Geometry: final body of the model. Coordinates: model frame, mm. A direction names the side the tool comes from. Coordinates: 2 decimals unless noted, no trailing zeros. Write each loop counter-clockwise with the first axis right and the second up, starting at its lowest first coordinate (ties: lowest second). Pieces come first, ordered by that corner, then holes. Notation, with made-up numbers: (11, 9.25) -> (48, 9.25) arc R20 cw to (48, 22.25) -> close; hole circle Ø11 at (10.5, -18.75). An arc over 180 degrees is marked (long way). One line per item, written item: value. Start each with the question number.
from build123d import *

# Parameters (mm, degrees)
F2_R    = 6
F3_SIZE = 1


with BuildPart() as f1:
    # F0 (on Front) → F1 (revolve)
    with BuildSketch(Plane.XZ):
        Polygon((-15.775755, -20), (-30.775755, -20), (-30.775755, -54.5), (-23.775755, -54.5), (-23.775755, -45), (-7.775755, -45), (-7.775755, -54.5), (2.224245, -54.5), (2.224245, -33), (7.224245, -33), (7.224245, -8), (2.224245, -8), (2.224245, -10.325), (-1.775755, -10.325), (-1.775755, -8), (-15.775755, -8), align=None)
    revolve(axis=Axis((-3.464836, 0, 0), (-1, 0, 0)))

    # F2
    f2_edges = [f1.edges().sort_by_distance(p)[0] for p in [
        (-30.775755, 0, 54.5),
    ]]
    fillet(f2_edges, radius=F2_R)

    # F3
    f3_edges = [f1.edges().sort_by_distance(p)[0] for p in [
        (-30.775755, 0, 20),
        (7.224245, 0, 8),
    ]]
    chamfer(f3_edges, length=F3_SIZE)


solid = f1.part
Q1. Cut plane A-A on x = -5. Output: boundary loops of the cut face in (y, z), and give its area (3 significant figures).
Q2. Cut plane B-B on x = -20.5. Output: boundary loops of the cut face in (y, z), and give its area (3 significant figures).
Q3. Access query for faces 4 (the flat face through (-15.776, 0, 9)), 5 (the flat face through (2.224, 23.5, -23.5)), 6 (the flat face through (2.224, 8, 3)), 7 (the cylindrical face through (4.2, 7.81, 1.73)), 8 (the flat face through (7.224, 7, -7)). Directions: +Z, -Z, +X, -X, +Y, -Y. A direction counts if a zero-diameter tool reaches every point of the face in a straight line with its end or side. Return the directions, or none.
Q4. Line query: L1, parallel to Z at x = -0.75, y = 0 (3 decimals); L2, parallel to X at y = -49, z = -0.5; L3, parallel to Z at x = -20.5, y = 0. Output: solid intervals per line, ascending. Write a range as from..to.
Q5. First-contact query: P1, Ø2, axis at x = -16, y = 38.5, coming from the -Z side; P2, Ø5, axis at y = -33, z = -18.5, coming from the +X side; P3, Ø2, axis at x = -24.5, z = 43, coming from the +Y side. Flat tips, straight axial feed; report the tip coordinate or a pass-through.
Q6. Draft query along Z for faces 1 (the cylindrical face through (-2.71, 33.16, 43.25)), 2 (the cylindrical face through (-22.874, 19.524, 4.336)), 3 (the flat face through (-30.776, 21, 10)). Return one class per face: pulls with the +Z half, pulls with the -Z half, needs draft (parallel to the pull), parting line crosses it, or undercut.
Solution:
1. outline: circle Ø109 at (0, 0); hole circle Ø16 at (0, 0)
1. area: 9,130 mm²
2. outline: circle Ø90 at (0, 0); hole circle Ø40 at (0, 0)
2. area: 5,110 mm²
3. face 4: -X
3. face 5: +X
3. face 6: none
3. face 7: +X, -X
3. face 8: +Z, -Z, +X, +Y, -Y
4. L1: -54.5..-10.325, 10.325..54.5
4. L2: -30.75..-23.78, -7.78..2.22
4. L3: -45..-20, 20..45
5. P1: z = -24.87
5. P2: x = 2.22
5. P3: y = 34.73
6. face 1: parting line crosses it
6. face 2: undercut
6. face 3: needs draft
